CAD build for the part. Positions are in the model's coordinates, mm. A direction names the side the tool comes from. Give positions to 0.01 mm unless a question says otherwise; leave off trailing zeros. Write each loop counter-clockwise with the first axis right and the second up, starting at its lowest first coordinate (ties: lowest second). Pieces come first, ordered by that corner, then holes. Notation, with made-up numbers: (14.5, 4) -> (38.5, 4) arc R23 cw to (38.5, 17) -> close; hole circle Ø6 at (13.5, 24). An arc over 180 degrees is marked (long way). Use one line per item in the form item = value. Start each with the question number.
from build123d import *

# Parameters (mm, degrees)
SKETCH_1_W      = 55
SKETCH_1_H      = 28
EXTRUDE_1_DEPTH = 1
SKETCH_2_W      = 15
SKETCH_2_H      = 15
EXTRUDE_2_DEPTH = 2
SKETCH_3_W      = 7
SKETCH_3_H      = 8
EXTRUDE_3_DEPTH = 2
FILLET_1_R      = 1


with BuildPart() as part:
    # 草图1 → 凸台-拉伸1 (new body)
    with BuildSketch(Plane.XY):
        Rectangle(SKETCH_1_W, SKETCH_1_H)
    extrude(amount=EXTRUDE_1_DEPTH)

    # 草图2 → 凸台-拉伸2 (add)
    with BuildSketch(Plane.XY.offset(1)):
        with Locations((17.5, 0)):
            Rectangle(SKETCH_2_W, SKETCH_2_H)
    extrude(amount=EXTRUDE_2_DEPTH)

    # 草图3 → 凸台-拉伸3 (add)
    with BuildSketch(Plane.XY.offset(1)):
        with Locations((-24, -7)):
            Rectangle(SKETCH_3_W, SKETCH_3_H)
        with Locations((-24, 7)):
            Rectangle(SKETCH_3_W, SKETCH_3_H)
    extrude(amount=EXTRUDE_3_DEPTH)

    # 圆角1
    fillet_1_edges = [part.edges().sort_by_distance(p)[0] for p in [
        (-24, 3, 3),
        (-24, 11, 3),
        (-24, -3, 3),
        (-24, -11, 3),
    ]]
    fillet(fillet_1_edges, radius=FILLET_1_R)


solid = part.part
1) 3-axis set-ups, long thin cutter, end or side, ignore diameter. For faces 1 (the face through (-24, 3, 1.5)), 2 (the face through (17, -7.5, 2)), 3 (the face through (17, 7.5, 2)), 4 (the face through (-24, -11, 1.5)), 5 (the face through (-20.5, -7, 2)): which of +Z, -Z, +X, -X, +Y, -Y reach the whole face in a straight line?
2) Cut at D-D (x = 15). Give the cut face in (y, z), and give its area (3 significant figures).
3) Pin check, flat tips, straight feed: pin 1 (0.6 mm diameter, centred on x = 20, z = 2, fed in from -Y); pin 2 (0.5 mm diameter, centred on x = -23.5, z = 1.5, fed in from +Y); pin 3 (1 mm diameter, centred on x = -7.5, y = -9, fed in from +Z). Stop position of each tip, or through.
4) Two-plate mould, pull along Y, no slides. Class faces 6 (the face through (-23.951, 3.285, 2.699)), 7 (the face through (-24, 11, 1.5)), 8 (the face through (17, 0, 3)): released by +Y, released by -Y, zero draft, split by the parting line, or undercut.
5) Cut at C-C (x = -23.5). Give the cut face in (y, z), and give its area (3 significant figures).
6) Cut at A-A (z = 1.5). Give the cut face in (x, y), and give its area (3 significant figures).
7) Cut at B-B (y = 6.25). Give the cut face in (x, z).
8) Wall check: line 1 along X through (y, z) = (4.5, 1.3); line 2 along Y through (x, z) = (-24.5, 1.8); line 3 along Z through (x, y) = (-15.5, -4.5). Give the ranges that are in metal, low to high. Write a range as from..to.
Final values:
q1.face_1 = +Z, -X
q1.face_2 = +Z, +X, -Y
q1.face_3 = +Z, +X, +Y
q1.face_4 = +Z, +X, -X, -Y
q1.face_5 = +Z, +Y, -Y
q2.outline = (-14, 0) -> (14, 0) -> (14, 1) -> (7.5, 1) -> (7.5, 3) -> (-7.5, 3) -> (-7.5, 1) -> (-14, 1) -> close
q2.area = 58.0 mm^2
q3.pin_1 = -7.5
q3.pin_2 = 11
q3.pin_3 = 1
q4.face_6 = undercut
q4.face_7 = released by +Y
q4.face_8 = zero draft
q5.outline = (-14, 0) -> (14, 0) -> (14, 1) -> (11, 1) -> (11, 2) arc R1 ccw to (10, 3) -> (4, 3) arc R1 ccw to (3, 2) -> (3, 1) -> (-3, 1) -> (-3, 2) arc R1 ccw to (-4, 3) -> (-10, 3) arc R1 ccw to (-11, 2) -> (-11, 1) -> (-14, 1) -> close
q5.area = 59.1 mm^2
q6.outline = (-27.5, -11) -> (-20.5, -11) -> (-20.5, -3) -> (-27.5, -3) -> close; (-27.5, 3) -> (-20.5, 3) -> (-20.5, 11) -> (-27.5, 11) -> close; (10, -7.5) -> (25, -7.5) -> (25, 7.5) -> (10, 7.5) -> close
q6.area = 337 mm^2
q7.outline = (-27.5, 0) -> (27.5, 0) -> (27.5, 1) -> (25, 1) -> (25, 3) -> (10, 3) -> (10, 1) -> (-20.5, 1) -> (-20.5, 3) -> (-27.5, 3) -> close
q8.line_1 = -27.5..-20.5, 10..25
q8.line_2 = -11..-3, 3..11
q8.line_3 = 0..1
